Build history of the part. All positions in model axes, mm. A direction names the side the tool comes from. Coordinates: 2 decimals unless noted, no trailing zeros. Order: outer loops, then holes, each group sorted by start corner. A loop starts at its lowest first (then second) coordinate and runs counter-clockwise, first axis right, second up. Notation, with made-up numbers: (39, -4.75) - (97, -4.75) arc R31 cw to (97, 29.25) - close; hole circle Ø9 at (60, 76.5). An arc over 180 degrees is marked (long way). Return JSON: item names as keys, results as strings.
from build123d import *

# Parameters (mm, degrees)
CHAMFER1_SIZE      = 0.3
CUT_EXTRUDE1_DEPTH = 2


with BuildPart() as part:
    # Sketch1 → Revolve1 (revolve)
    with BuildSketch(Plane.XY, mode=Mode.PRIVATE) as revolve1_sk:
        Polygon((5, 3), (6, 2), (6, 0), (0, 0), (0, 3), align=None)
    revolve(revolve1_sk.sketch.rotate(Axis((0, 0, 0), (1, 0, 0)), 90), axis=Axis((0, 0, 0), (1, 0, 0)))

    # Chamfer1
    chamfer1_edges = [part.edges().sort_by_distance(p)[0] for p in [
        (0, 0, -3),
    ]]
    chamfer(chamfer1_edges, length=CHAMFER1_SIZE)

    # Sketch2 → Cut-Extrude1 (cut)
    with BuildSketch(Plane(origin=(0, 0, 0), x_dir=(0, 0, -1), z_dir=(1, 0, 0))):
        Polygon((0, 1.732050808), (-1.5, 0.866025404), (-1.5, -0.866025404), (0, -1.732050808), (1.5, -0.866025404), (1.5, 0.866025404), align=None)
    extrude(amount=CUT_EXTRUDE1_DEPTH, mode=Mode.SUBTRACT)

    # Sketch3 → Cut-Revolve1 (revolve, cut)
    with BuildSketch(Plane.XY, mode=Mode.PRIVATE) as cut_revolve1_sk:
        Polygon((2.866025404, 0), (2, 1.5), (2, 0), align=None)
    revolve(cut_revolve1_sk.sketch.rotate(Axis((2, 0, 0), (1, 0, 0)), 270), axis=Axis((2, 0, 0), (1, 0, 0)), mode=Mode.SUBTRACT)


solid = part.part
1. Probe L1, parallel to Y at x = 1.6, z = 0.6; L2, parallel to Y at x = 1.2, z = 1.3; L3, parallel to Z at x = 0.4, y = -1.6. List the from-to ranges inside material, lowest first.
Check values:
{"L1": "-2.94 to -1.39, 1.39 to 2.94", "L2": "-2.7 to -0.98, 0.98 to 2.7", "L3": "-2.54 to -0.23, 0.23 to 2.54"}
2. Cut at A-A on x = 1.9. Give the cut face in (y, z).
Check values:
{"outline": "circle Ø6 at (0, 0); hole (-1.73, 0) - (-0.87, -1.5) - (0.87, -1.5) - (1.73, 0) - (0.87, 1.5) - (-0.87, 1.5) - close"}
3. Cut at B-B on x = 3.6. Give the cut face in (y, z), plus the area to 3 significant figures.
Check values:
{"outline": "circle Ø6 at (0, 0)", "area": "28.3 mm²"}
4. Tool access for faces 4 (the flat face through (1, 0, 1.5)), 5 (the flat face through (6, 0, 0)): list every direction of +Z, -Z, +X, -X, +Y, -Y with a clear straight run to the whole face (end or side of a thin tool).
Check values:
{"face 4": "-X", "face 5": "+Z, -Z, +X, +Y, -Y"}
5. Mould opens along Y. For faces 1 (the conical face through (2.716, -0.231, -0.12)), 2 (the cylindrical face through (2.68, -0.9, 2.86)), 3 (the flat face through (0, 2, 0)) say: pulls with the +Y half, pulls with the -Y half, needs draft (parallel to the pull), parting line crosses it, or undercut.
Check values:
{"face 1": "undercut", "face 2": "parting line crosses it", "face 3": "needs draft"}
6. Drop flat-ended pins along their axis: pin 1 (0.9 mm diameter, centred on x = 0.5, y = -0.5, fed in from +Z); pin 2 (1.5 mm diameter, centred on x = 5.5, z = -1.5, fed in from +Y). Give the stop position or say it passes through.
Check values:
{"pin 1": "z = 3", "pin 2": "y = 2.85"}
